Geometry: final body of the model. Coordinates: model frame, mm. Coordinates: 2 decimals unless noted, no trailing zeros. Loops run counter-clockwise (first coordinate to the right, second up) from the corner with the lowest first, then second, coordinate; pieces in that order, holes last. Notation, with made-up numbers: (69.25, 78.5) - (112.25, 78.5) arc R13 cw to (112.25, 98.5) - close; hole circle Ø5 at (23.5, -31.5). An arc over 180 degrees is marked (long way). Answer in a Markdown table with one row per item.
from build123d import *

# Parameters (mm, degrees)
SALIENTE_EXTRUIR1_DEPTH = 0.1


with BuildPart() as part:
    # Model → Saliente-Extruir1 (new body)
    with BuildSketch(Plane.XY):
        with BuildLine():
            Line((12.698297287, 13.802618595), (15.263616387, 13.750921574))
            ThreePointArc((15.263616387, 13.750921574), (14.654945019, 9.542094065), (15.782845256, 5.441782991))
            ThreePointArc((15.782845256, 5.441782991), (17.35183527, 2.94274106), (18.745376573, 0.341782991))
            ThreePointArc((18.745376573, 0.341782991), (19.372340085, -1.579426143), (19.782845256, -3.558217009))
            Line((19.782845256, -3.558217009), (21.782845256, -2.558217009))
            ThreePointArc((21.782845256, -2.558217009), (21.595097776, -1.089252971), (21.213993411, 0.341782991))
            ThreePointArc((21.213993411, 0.341782991), (19.656131166, 2.997887435), (17.782845256, 5.441782991))
            ThreePointArc((17.782845256, 5.441782991), (16.97662621, 6.680138732), (16.643698969, 8.119817009))
            Line((16.643698969, 8.119817009), (16.284102713, 8.119817009))
            Line((16.284102713, 8.119817009), (16.284102713, 16.741782991))
            Line((16.284102713, 16.741782991), (12.782845256, 16.741782991))
            Line((12.782845256, 16.741782991), (12.698297287, 13.802618595))
        make_face()
    extrude(amount=SALIENTE_EXTRUIR1_DEPTH)


solid = part.part
(1) Cut plane C-C on x = 14. Output: boundary loops of the cut face in (y, z), then the cut area to 3 significant figures.
Verdict:
| item | result |
|---|---|
| outline | (13.78, 0) - (16.74, 0) - (16.74, 0.1) - (13.78, 0.1) - close |
| area | 0.297 mm² |
(2) Cut plane B-B on y = 3. Output: boundary loops of the cut face in (x, z).
Verdict:
| item | result |
|---|---|
| outline | (17.32, 0) - (19.65, 0) - (19.65, 0.1) - (17.32, 0.1) - close |
(3) Ray query, probe 1 along Y at (x, z) = (14, 0.05); probe 2 along X at (y, z) = (14.25, 0.05); probe 3 along Y at (x, z) = (17.75, 0.05). Return the intervals inside material, ascending.
Verdict:
| item | result |
|---|---|
| probe 1 | y = 13.78 to 16.74 |
| probe 2 | x = 12.71 to 16.28 |
| probe 3 | y = 2.24 to 5.48 |
(4) Cut plane A-A on z = 0.05. Output: boundary loops of the cut face in (x, y).
Verdict:
| item | result |
|---|---|
| outline | (12.7, 13.8) - (15.26, 13.75) arc R10.39 ccw to (15.78, 5.44) arc R42.91 cw to (18.75, 0.34) arc R18.23 cw to (19.78, -3.56) - (21.78, -2.56) arc R11.13 ccw to (21.21, 0.34) arc R24.94 ccw to (17.78, 5.44) arc R4.25 cw to (16.64, 8.12) - (16.28, 8.12) - (16.28, 16.74) - (12.78, 16.74) - close |
